Here's how the part is built. I have some questions about the finished solid (model axes, mm). Give positions to 0.01 mm unless a question says otherwise; leave off trailing zeros. Loops run counter-clockwise (first coordinate to the right, second up) from the corner with the lowest first, then second, coordinate; pieces in that order, holes last. Notation, with made-up numbers: (18.5, 64.5) - (77.5, 64.5) arc R21 ccw to (77.5, 78.5) - close; hole circle Ø6 at (72.25, 60.25). An arc over 180 degrees is marked (long way). Use one line per item in the form item = value.
from build123d import *

# Parameters (mm, degrees)
F0_R     = 36
F0_R_2   = 11
F1_DEPTH = 17.5
F2_R     = 10
F3_SIZE  = 5


with BuildPart() as f1:
    # F0 (on Front) → F1 (new body, symmetric)
    with BuildSketch(Plane.XZ):
        Circle(F0_R)
        Circle(F0_R_2, mode=Mode.SUBTRACT)
    extrude(amount=F1_DEPTH, both=True)

    # F2
    f2_edges = [f1.edges().sort_by_distance(p)[0] for p in [
        (-36, -17.5, 0),
        (-36, 17.5, 0),
    ]]
    fillet(f2_edges, radius=F2_R)

    # F3
    f3_edges = [f1.edges().sort_by_distance(p)[0] for p in [
        (36, 0, 0),
        (-36, 7.5, 0),
        (-36, -7.5, 0),
        (-11, -17.5, 0),
        (-11, 17.5, 0),
    ]]
    chamfer(f3_edges, length=F3_SIZE)


solid = f1.part
(1) If we section it at C-C (y = -4): List the corners of the cut face in (x, z) for me, plus the area to 3 significant figures.
Geometry says:
outline = circle Ø72 at (0, 0); hole circle Ø22 at (0, 0)
area = 3,690 mm²
(2) For P1, Ø10, axis at x = -9, z = -3.5, coming from the +Y side; P2, Ø2, axis at y = -6.5, z = -24, coming from the -X side; P3, Ø1.5, axis at x = 21.5, y = -8.5, coming from the -Z side; P4, Ø4, axis at x = 12, z = 10.5, coming from the +Y side, each with a flat end and sliding along its axis, tell me the tip position at first contact or that it passes through.
Geometry says:
P1 = 16.16
P2 = -27.69
P3 = -29.36
P4 = 17.5
(3) If we section it at B-B (x = 0): List the corners of the cut face in (y, z) for me, plus the area to 3 significant figures.
Geometry says:
outline = (-17.5, -26) arc R10 ccw to (-7.5, -36) - (7.5, -36) arc R10 ccw to (17.5, -26) - (17.5, -16) - (12.5, -11) - (-12.5, -11) - (-17.5, -16) - close; (-17.5, 16) - (-12.5, 11) - (12.5, 11) - (17.5, 16) - (17.5, 26) arc R10 ccw to (7.5, 36) - (-7.5, 36) arc R10 ccw to (-17.5, 26) - close
area = 1,610 mm²
(4) If I drill on probe 1 along Z at (x, y) = (0, -6); probe 2 along Z at (x, y) = (1.5, -9); probe 3 along X at (y, z) = (4.5, 8), over which ranges is the centre line in solid material (lowest first)?
Geometry says:
probe_1 = -36 to -11, 11 to 36
probe_2 = -35.86 to -10.9, 10.9 to 35.86
probe_3 = -35.1 to -7.55, 7.55 to 35.1
(5) Thinking about a two-plate mould opening in X: for faces 1 (the cylindrical face through (-4.686, -0.105, 35.694)), 2 (the cylindrical face through (-2.38, 0.18, -10.74)), 3 (the flat face through (11, 17.5, 12)), 4 (the conical face through (-2.437, -12.743, -10.975)), which applies, pulls with the +X half, pulls with the -X half, needs draft (parallel to the pull), parting line crosses it, or undercut?
Geometry says:
face_1 = parting line crosses it
face_2 = undercut
face_3 = needs draft
face_4 = undercut
(6) If we section it at A-A (z = 0): List the corners of the cut face in (x, y) for me, plus the area to 3 significant figures.
Geometry says:
outline = (-36, -7.5) arc R10 ccw to (-26, -17.5) - (-16, -17.5) - (-11, -12.5) - (-11, 12.5) - (-16, 17.5) - (-26, 17.5) arc R10 ccw to (-36, 7.5) - close; (11, -12.5) - (16, -17.5) - (26, -17.5) arc R10 ccw to (36, -7.5) - (36, 7.5) arc R10 ccw to (26, 17.5) - (16, 17.5) - (11, 12.5) - close
area = 1,610 mm²
